Build history of the part. All positions in model axes, mm. Face numbers are marked on the shaded views. A direction names the side the tool comes from. Round coordinates to 2 decimals unless told otherwise and drop trailing zeros. Write each loop counter-clockwise with the first axis right and the second up, starting at its lowest first coordinate (ties: lowest second). Pieces come first, ordered by that corner, then holes. Notation, with made-up numbers: M 4,66.25 L 58,66.25 A7 cw 58,78.25 Z; hole C 48.5,46 d6. An arc over 180 degrees is marked long. Write item = value, one per line. Start each with the question number.
Q1. Tool access for the marked faces 1, 2, 3 and 4: list every direction of +Z, -Z, +X, -X, +Y, -Y with a clear straight run to the whole face (end or side of a thin tool).
Q2. Pull direction X, two halves, no side cores. Call the marked faces 5, 6, 7 and 8: released by +X, released by -X, zero draft, split by the parting line, or undercut.
Q3. Band-saw the part on C-C on y = 6. Write the cut outline in (x, z).
Q4. Band-saw the part on A-A on z = 45.5. Write the cut outline in (x, y), plus the area to 3 significant figures.
Q5. Probe L1, parallel to X at y = -9.5, z = 43.5; L2, parallel to Y at x = 15.8, z = 42.5; L3, parallel to Z at x = 6.5, y = -9. List the from-to ranges inside material, lowest first.
Q6. Band-saw the part on B-B on z = 34.5. Write the cut outline in (x, y), plus the area to 3 significant figures.
Q7. Band-saw the part on D-D on z = 8. Write the cut outline in (x, y), plus the area to 3 significant figures.
Q8. Drop flat-ended pins along their axis: P1, Ø6.5, axis at x = -16.5, z = 42, coming from the -Y side; P2, Ø6, axis at y = 2, z = 19, coming from the +X side; P3, Ø0.5, axis at x = -6.5, y = -1.5, coming from the -Z side. Give the stop position or say it passes through.
```python
from build123d import *

# Parameters (mm, degrees)
BOSS_EXTRUDE1_DEPTH      = 20
BOSS_EXTRUDE2_DEPTH      = 11
BOSS_EXTRUDE2_DEPTH_BACK = 11
CUT_EXTRUDE1_DEPTH       = 63.171134781
CUT_EXTRUDE1_DEPTH_BACK  = 63.171134781
SKETCH3_R                = 5
SKETCH3_R_2              = 4.5


with BuildPart() as part:
    # Sketch1 → Boss-Extrude1 (new body)
    with BuildSketch(Plane.XY):
        with BuildLine():
            Line((-12, -18), (-12, 0))
            ThreePointArc((-12, 0), (0, 12), (12, 0))
            Line((12, 0), (12, -18))
            ThreePointArc((12, -18), (7, -23), (2, -18))
            Line((2, -18), (2, -6.708203932))
            ThreePointArc((2, -6.708203932), (0, 7), (-2, -6.708203932))
            Line((-2, -6.708203932), (-2, -18))
            ThreePointArc((-2, -18), (-7, -23), (-12, -18))
        make_face()
    extrude(amount=BOSS_EXTRUDE1_DEPTH)

    # Sketch2 → Boss-Extrude2 (add, two sides: drawn at the far end of the back side and taken through both)
    with BuildSketch(Plane(origin=(0, 0, 0), x_dir=(1, 0, 0), z_dir=(0, 1, 0)).offset(-BOSS_EXTRUDE2_DEPTH_BACK)):
        with BuildLine():
            Line((-20.5, -51), (-20.5, -24))
            ThreePointArc((-20.5, -24), (-18.075652903, -17.540680891), (-12, -14.271628429))
            Line((-12, -14.271628429), (-5.296851039, -14.271628429))
            Line((-5.296851039, -14.271628429), (-5.296851039, -20))
            ThreePointArc((-5.296851039, -20), (-11.707630257, -21.787067507), (-14.5, -27.828124672))
            Line((-14.5, -27.828124672), (-14.5, -51))
            ThreePointArc((-14.5, -51), (-17.5, -54), (-20.5, -51))
        make_face()
        with BuildLine():
            Line((14.5, -51), (14.5, -27.828124672))
            ThreePointArc((14.5, -27.828124672), (11.707630257, -21.787067507), (5.296851039, -20))
            Line((5.296851039, -20), (5.296851039, -14.271628429))
            Line((5.296851039, -14.271628429), (12, -14.271628429))
            ThreePointArc((12, -14.271628429), (18.075652903, -17.540680891), (20.5, -24))
            Line((20.5, -24), (20.5, -51))
            ThreePointArc((20.5, -51), (17.5, -54), (14.5, -51))
        make_face()
    extrude(amount=BOSS_EXTRUDE2_DEPTH + BOSS_EXTRUDE2_DEPTH_BACK)

    # Sketch3 → Cut-Extrude1 (cut, two sides: drawn at the far end of the back side and taken through both)
    with BuildSketch(Plane(origin=(0, 0, 0), x_dir=(0, 0, -1), z_dir=(1, 0, 0)).offset(-CUT_EXTRUDE1_DEPTH_BACK)):
        with Locations((-42.5, 0)):
            Circle(SKETCH3_R)
        with Locations((-8, -9)):
            Circle(SKETCH3_R_2)
    extrude(amount=CUT_EXTRUDE1_DEPTH + CUT_EXTRUDE1_DEPTH_BACK, mode=Mode.SUBTRACT)


solid = part.part
```
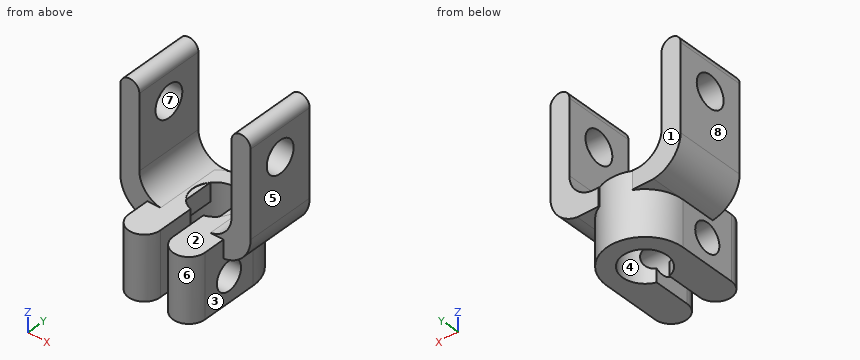
Conclusion:
q1.face_1 = +Z, -Z, -X, +Y
q1.face_2 = +Z, -Y
q1.face_3 = -Z, +X, -Y
q1.face_4 = -Z
q2.face_5 = released by +X
q2.face_6 = undercut
q2.face_7 = zero draft
q2.face_8 = released by -X
q3.outline = M -20.5,24 A9.82 ccw -12,14.27 L -10.39,14.27 L -10.39,0 L -3.61,0 L -3.61,20 L -7.84,20 A7.93 cw -14.5,27.83 L -14.5,51 A3 ccw -20.5,51 Z; M 3.61,0 L 10.39,0 L 10.39,14.27 L 12,14.27 A9.82 ccw 20.5,24 L 20.5,51 A3 ccw 14.5,51 L 14.5,27.83 A7.93 cw 7.84,20 L 3.61,20 Z
q4.outline = M -20.5,-11 L -14.5,-11 L -14.5,-4 L -20.5,-4 Z; M -20.5,4 L -14.5,4 L -14.5,11 L -20.5,11 Z; M 14.5,-11 L 20.5,-11 L 20.5,-4 L 14.5,-4 Z; M 14.5,4 L 20.5,4 L 20.5,11 L 14.5,11 Z
q4.area = 168 mm^2
q5.L1 = -20.5 to -14.5, 14.5 to 20.5
q5.L2 = -11 to -5, 5 to 11
q5.L3 = 0 to 3.5, 12.5 to 20
q6.outline = M -20.5,-11 L -14.5,-11 L -14.5,11 L -20.5,11 Z; M 14.5,-11 L 20.5,-11 L 20.5,11 L 14.5,11 Z
q6.area = 264 mm^2
q7.outline = M -12,-18 A5 ccw -2,-18 L -2,-13.5 L -12,-13.5 Z; M -12,-4.5 L -5.36,-4.5 A7 cw long 5.36,-4.5 L 12,-4.5 L 12,0 A12 ccw -12,0 Z; M 2,-18 A5 ccw 12,-18 L 12,-13.5 L 2,-13.5 Z
q7.area = 367 mm^2
q8.P1 = -11
q8.P2 = 20.29
q8.P3 = 14.27
